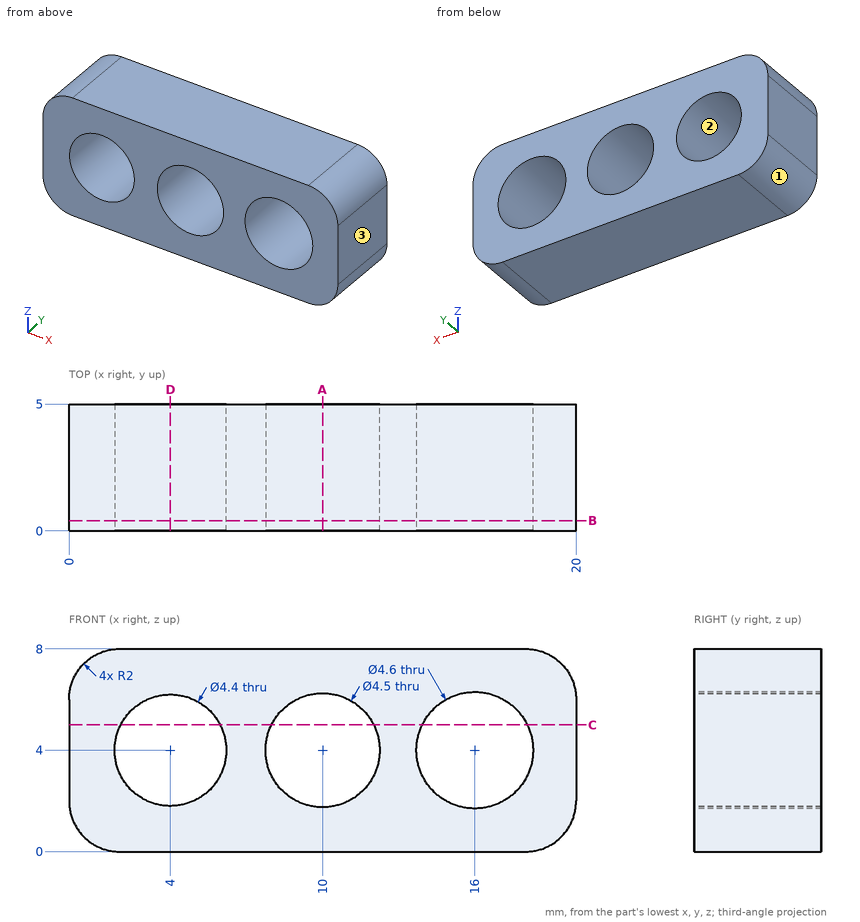
Print and shaded views of the part. All mm, measured from the part's lowest x, y and z. Give positions to 0.01 mm unless a question says otherwise; leave off trailing zeros. Loops run counter-clockwise (first coordinate to the right, second up) from the corner with the lowest first, then second, coordinate; pieces in that order, holes last. Notation, with made-up numbers: (27.5, 77.25) -> (80.5, 77.25) arc R32 cw to (80.5, 113.25) -> close; hole circle Ø8 at (-19, -20). An arc over 180 degrees is marked (long way). One line per question, with ' | ' between items. Start each with the question number.
1) Cut at D-D (x = 4). Give the cut face in (y, z).
2) Cut at A-A (x = 10). Give the cut face in (y, z).
3) Two-plate mould, pull along Z, no slides. Class the marked faces 1, 2 and 3: released by +Z, released by -Z, zero draft, split by the parting line, or undercut.
4) Cut at B-B (y = 0.4). Give the cut face in (x, z).
5) Probe L1, parallel to X at y = 1.45, z = 4; L2, parallel to Z at x = 10, y = 3.85; L3, parallel to Z at x = 16, y = 3.9. List the from-to ranges inside material, lowest first.
6) Cut at C-C (z = 5). Give the cut face in (x, y), plus the area to 3 significant figures.
Return value:
1) outline: (0, 0) -> (5, 0) -> (5, 1.8) -> (0, 1.8) -> close; (0, 6.2) -> (5, 6.2) -> (5, 8) -> (0, 8) -> close
2) outline: (0, 0) -> (5, 0) -> (5, 1.75) -> (0, 1.75) -> close; (0, 6.25) -> (5, 6.25) -> (5, 8) -> (0, 8) -> close
3) face 1: released by -Z | face 2: undercut | face 3: zero draft
4) outline: (0, 2) arc R2 ccw to (2, 0) -> (18, 0) arc R2 ccw to (20, 2) -> (20, 6) arc R2 ccw to (18, 8) -> (2, 8) arc R2 ccw to (0, 6) -> close; hole circle Ø4.4 at (4, 4); hole circle Ø4.5 at (10, 4); hole circle Ø4.6 at (16, 4)
5) L1: 0 to 1.8, 6.2 to 7.75, 12.25 to 13.7, 18.3 to 20 | L2: 0 to 1.75, 6.25 to 8 | L3: 0 to 1.7, 6.3 to 8
6) outline: (0, 0) -> (2.04, 0) -> (2.04, 5) -> (0, 5) -> close; (5.96, 0) -> (7.98, 0) -> (7.98, 5) -> (5.96, 5) -> close; (12.02, 0) -> (13.93, 0) -> (13.93, 5) -> (12.02, 5) -> close; (18.07, 0) -> (20, 0) -> (20, 5) -> (18.07, 5) -> close | area: 39.5 mm^2
